Could you check a few things on this model? Use its own coordinates, in mm. Face numbers are marked on the shaded views. A direction names the side the tool comes from. Coordinates: 2 decimals unless noted, no trailing zeros. Order: outer loops, then holes, each group sorted by start corner. A loop starts at its lowest first (then second) coordinate and runs counter-clockwise, first axis right, second up. Notation, with made-up numbers: (-20.5, 83) -> (3.5, 83) arc R25 cw to (3.5, 108) -> close; hole circle Ø1 at (86, 18.25). An arc over 180 degrees is marked (long way). Put each result on its own line as item: value. Start each with the question number.
Q1. We'd pull the mould along Y, two halves only. Please class the marked faces 1, 2, 3 and 4: +Y half, -Y half, draft (parallel to the pull), parting line (faces both ways), or undercut.
Q2. Will this pin go through, and if not, where does the flat tip stop? pin 1 (6 mm diameter, centred on x = -12.5, y = 21, fed in from +Z).
Q3. Please list where these lines run through material, in increasing order: line 1 along X through (y, z) = (-63.5, 12.75) (3 decimals); line 2 along Y through (x, z) = (-26.5, 11) (3 decimals); line 3 along X through (y, z) = (27.5, 15.25) (3 decimals).
Q4. If we section it at B-B (y = 31): Please give me the cut outline in (x, z) (3 decimals).
Q5. If we section it at A-A (z = 11.5): Please give me the cut outline in (x, y) (3 decimals), and give its area (3 significant figures).
Q6. For the marked faces 5 and 6, which set-ups out of +Z, -Z, +X, -X, +Y, -Y let a thin tool reach every point of the face, with its end or its side?
Q7. If we section it at C-C (x = 20.5): Please give me the cut outline in (y, z) (3 decimals), and give its area (3 significant figures).
from build123d import *

# Parameters (mm, degrees)
F0_W     = 63.5
F0_H     = 146.05
F1_DEPTH = 25.4
F2_W     = 57.15
F2_H     = 133.35
F3_DEPTH = 19.05
F4_R     = 0.898026
F4_R_2   = 1.27
F4_R_3   = 1.881193
F4_R_4   = 1.948089
F5_DEPTH = 19.05
F6_R     = 2.54


with BuildPart() as f1:
    # F0 (on Top) → F1 (new body)
    with BuildSketch(Plane.XY):
        Rectangle(F0_W, F0_H)
    extrude(amount=F1_DEPTH)

    # F2 (on face) → F3 (cut)
    with BuildSketch(Plane.XY.offset(25.4)):
        Rectangle(F2_W, F2_H)
    extrude(amount=-F3_DEPTH, mode=Mode.SUBTRACT)

    # F4 (on face) → F5 (join)
    with BuildSketch(Plane.XY.offset(6.35)):
        with Locations((-6.438811, 27.302402)):
            Circle(F4_R)
        with Locations((3.009427, 27.399807)):
            Circle(F4_R_2)
        with Locations((-7.218048, 5.970811)):
            Circle(F4_R_3)
        with Locations((3.788662, 6.652642)):
            Circle(F4_R_4)
    extrude(amount=F5_DEPTH)

    # F6
    f6_edges = [f1.edges().sort_by_distance(p)[0] for p in [
        (-31.75, -73.025, 12.7),
        (31.75, -73.025, 12.7),
        (0, -73.025, 0),
        (0, -73.025, 25.4),
    ]]
    fillet(f6_edges, radius=F6_R)


solid = f1.part
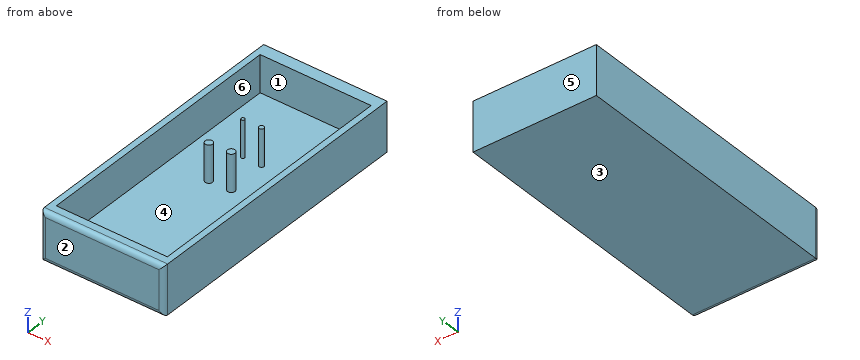
The answers:
1. face 1: undercut
1. face 2: -Y half
1. face 3: draft
1. face 4: undercut
2. pin 1: z = 6.35
3. line 1: -31.75 to -28.575, 28.575 to 31.75
3. line 2: -73.025 to -66.675, 66.675 to 73.025
3. line 3: -31.75 to -28.575, -7.315 to -5.563, 1.743 to 4.275, 28.575 to 31.75
4. outline: (-31.75, 0) -> (31.75, 0) -> (31.75, 25.4) -> (28.575, 25.4) -> (28.575, 6.35) -> (-28.575, 6.35) -> (-28.575, 25.4) -> (-31.75, 25.4) -> close
5. outline: (-31.75, -70.485) arc R2.54 ccw to (-29.21, -73.025) -> (29.21, -73.025) arc R2.54 ccw to (31.75, -70.485) -> (31.75, 73.025) -> (-31.75, 73.025) -> close; circle Ø3.762 at (-7.218, 5.971); circle Ø1.796 at (-6.439, 27.302); circle Ø2.54 at (3.009, 27.4); circle Ø3.896 at (3.789, 6.653); hole (-28.575, -66.675) -> (28.575, -66.675) -> (28.575, 66.675) -> (-28.575, 66.675) -> close
5. area: 1,680 mm^2
6. face 5: +Z, -Z, +X, -X, +Y
6. face 6: +Z
7. outline: (-73.025, 2.54) arc R2.54 ccw to (-70.485, 0) -> (73.025, 0) -> (73.025, 25.4) -> (66.675, 25.4) -> (66.675, 6.35) -> (-66.675, 6.35) -> (-66.675, 25.4) -> (-70.485, 25.4) arc R2.54 ccw to (-73.025, 22.86) -> close
7. area: 1,170 mm^2
